Build history of the part. All positions in model axes, mm. A direction names the side the tool comes from. Give positions to 0.01 mm unless a question says otherwise; leave off trailing zeros. Write each loop counter-clockwise with the first axis right and the second up, starting at its lowest first coordinate (ties: lowest second). Pieces come first, ordered by that corner, then holes. Notation, with made-up numbers: (35, 71) -> (73, 71) arc R20 ccw to (73, 108) -> close; hole circle Ø6 at (2.25, -5). An arc over 180 degrees is marked (long way). One line per question, with ' | ' between items. Start each with the question number.
(1) Tool access for faces 5 (the flat face through (0, 14, -2)), 6 (the flat face through (0, 3, 6)), 7 (the cylindrical face through (0.1, 14.4, -6.5)), 8 (the flat face through (5, -5, 0)), 9 (the cylindrical face through (-0.1, 14.4, 6.5)): list every direction of +Z, -Z, +X, -X, +Y, -Y with a clear straight run to the whole face (end or side of a thin tool).
(2) Band-saw the part on B-B, the plane x = 2.5. Give the cut face in (y, z).
(3) Pull direction Z, two halves, no side cores. Call faces 1 (the flat face through (4.58, 7.73, 10.37)), 2 (the flat face through (0, 19.5, -4)), 3 (the flat face through (0, 14, 2)), 4 (the flat face through (4.094, 7.726, -10.573)): released by +Z, released by -Z, zero draft, split by the parting line, or undercut.
(4) Band-saw the part on C-C, the plane y = 16.25. Give the cut face in (x, z), and give its area (3 significant figures).
(5) Band-saw the part on A-A, the plane z = 3.75. Give the cut face in (x, y), and give its area (3 significant figures).
(6) Band-saw the part on D-D, the plane y = -3.5. Give the cut face in (x, z), and give its area (3 significant figures).
(7) Drill centre lines: probe 1 along Y at (x, z) = (7.75, -8.25); probe 2 along Z at (x, y) = (-1.25, -8.5); probe 3 along Y at (x, z) = (1.5, -1). Where is each one in solid material? Low to high. Write a range as from..to.
(8) Pin check, flat tips, straight feed: P1, Ø5, axis at y = -4.5, z = 0.5, coming from the -X side; P2, Ø3, axis at x = 0.5, y = 4, coming from the -Z side; P3, Ø1.5, axis at x = -2.5, y = 10.5, coming from the +Z side. Stop position of each tip, or through.
from build123d import *

# Parameters (mm, degrees)
SKETCH1_W            = 10
SKETCH1_H            = 10
BOSS_EXTRUDE1_DEPTH  = 10
SKETCH2_W            = 12
SKETCH2_H            = 12
BOSS_EXTRUDE5_DEPTH  = 6
BOSS_EXTRUDE6_DEPTH  = 3.5
BOSS_EXTRUDE11_DEPTH = 10


with BuildPart() as part:
    # Sketch1 → Boss-Extrude1 (new body)
    with BuildSketch(Plane(origin=(0, 0, 0), x_dir=(1, 0, 0), z_dir=(0, 1, 0))):
        Rectangle(SKETCH1_W, SKETCH1_H)
    extrude(amount=-BOSS_EXTRUDE1_DEPTH)

    # Sketch2 → Boss-Extrude5 (add)
    with BuildSketch(Plane(origin=(0, 0, 0), x_dir=(1, 0, 0), z_dir=(0, 1, 0))):
        Rectangle(SKETCH2_W, SKETCH2_H)
    extrude(amount=BOSS_EXTRUDE5_DEPTH)

    # Sketch4 → Boss-Extrude6 (add)
    with BuildSketch(Plane(origin=(0, 6, 0), x_dir=(1, 0, 0), z_dir=(0, 1, 0))):
        Polygon((0.35623678, -12.266936068), (8.925931121, -8.422136236), (12.266936068, 0.35623678), (8.422136236, 8.925931121), (-0.35623678, 12.266936068), (-8.925931121, 8.422136236), (-12.266936068, -0.35623678), (-8.422136236, -8.925931121), align=None)
    extrude(amount=BOSS_EXTRUDE6_DEPTH)

    # Sketch8 → Boss-Extrude11 (add)
    with BuildSketch(Plane(origin=(0, 9.5, 0), x_dir=(1, 0, 0), z_dir=(0, 1, 0))):
        with BuildLine():
            Line((-6.184658438, 2), (6.184658438, 2))
            ThreePointArc((6.184658438, 2), (0, 6.5), (-6.184658438, 2))
        make_face()
        with BuildLine():
            Line((6.184658438, -2), (-6.184658438, -2))
            ThreePointArc((-6.184658438, -2), (0, -6.5), (6.184658438, -2))
        make_face()
    extrude(amount=BOSS_EXTRUDE11_DEPTH)


solid = part.part
Results:
1) face 5: +X, -X, +Y | face 6: +Z, +X, -X, -Y | face 7: -Z, +Y | face 8: +Z, -Z, +X, -Y | face 9: +Z, +Y
2) outline: (-10, -5) -> (0, -5) -> (0, -6) -> (6, -6) -> (6, -11.18) -> (9.5, -11.18) -> (9.5, -6) -> (19.5, -6) -> (19.5, -2) -> (9.5, -2) -> (9.5, 2) -> (19.5, 2) -> (19.5, 6) -> (9.5, 6) -> (9.5, 11.31) -> (6, 11.31) -> (6, 6) -> (0, 6) -> (0, 5) -> (-10, 5) -> close
3) face 1: released by +Z | face 2: zero draft | face 3: undercut | face 4: released by -Z
4) outline: (-6.18, -2) arc R6.5 ccw to (6.18, -2) -> close; (-6.18, 2) -> (6.18, 2) arc R6.5 ccw to start | area: 81.6 mm²
5) outline: (-10.74, 6) -> (-6, 6) -> (-6, 0) -> (-5, 0) -> (-5, -10) -> (5, -10) -> (5, 0) -> (6, 0) -> (6, 6) -> (10.7, 6) -> (10.7, 9.5) -> (5.31, 9.5) -> (5.31, 19.5) -> (-5.31, 19.5) -> (-5.31, 9.5) -> (-10.74, 9.5) -> close | area: 353 mm²
6) outline: (-5, -5) -> (5, -5) -> (5, 5) -> (-5, 5) -> close | area: 100 mm²
7) probe 1: y = 6..9.5 | probe 2: z = -5..5 | probe 3: y = -10..9.5
8) P1: stops at x = -5 | P2: stops at z = -6 | P3: stops at z = 6.26
